The drawing under review shows one solid part. Ordinate dimensions are in mm from its lowest x, y, z. A direction names the side the tool comes from. Coordinates: 2 decimals unless noted, no trailing zeros. Loops run counter-clockwise (first coordinate to the right, second up) from the corner with the lowest first, then second, coordinate; pieces in that order, holes last. Notation, with made-up numbers: M 65.25,-13.5 L 88.25,-13.5 A17 cw 88.25,-0.5 Z; hole C 65,39 d9. An arc over 180 degrees is marked long. Put each result on its own line as item: value.
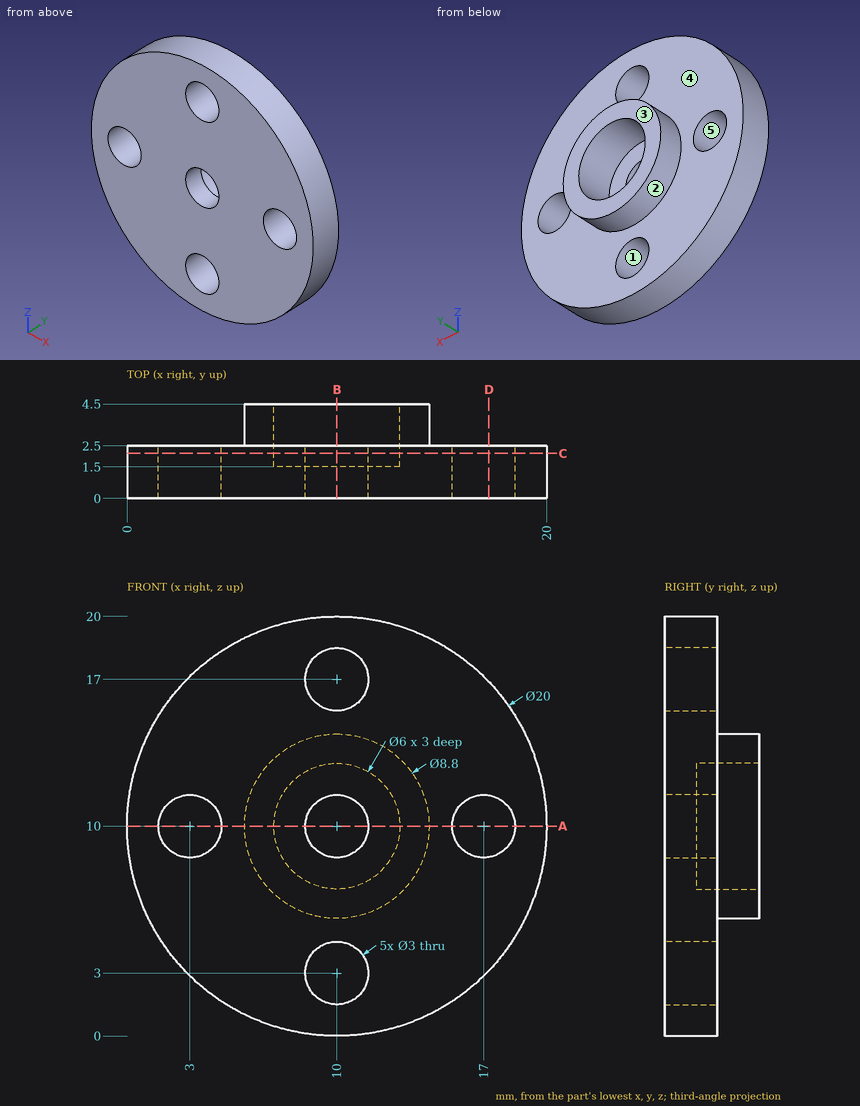
(1) Add section D-D (x = 17.25). Write out the cut boundary in (y, z).
Determined:
outline: M 0,3.11 L 2.5,3.11 L 2.5,8.52 L 0,8.52 Z; M 0,11.48 L 2.5,11.48 L 2.5,16.89 L 0,16.89 Z
(2) Tool access review of the marked faces 4 and 5: name each direction out of +Z, -Z, +X, -X, +Y, -Y from which nothing blocks a thin tool from reaching the whole face with its end or side.
Determined:
face 4: +Y
face 5: +Y, -Y
(3) For pin 1 (4 mm diameter, centred on x = 10, z = 17, fed in from +Y); pin 2 (1.5 mm diameter, centred on y = 1.5, z = 13.5, fed in from -X); pin 3 (2 mm diameter, centred on y = 1, z = 16, fed in from -X), all flat-tipped, find the tip position at first contact; note any pin that passes through.
Determined:
pin 1: stops at y = 2.5
pin 2: stops at x = 0.39
pin 3: stops at x = 1.34
(4) Draft analysis for pull direction Z (two halves, no side actions). For the marked faces 1, 2 and 3, state which applies: +Z half, -Z half, draft (parallel to the pull), parting line (faces both ways), or undercut.
Determined:
face 1: undercut
face 2: parting line
face 3: draft
(5) Wall thickness on line 1 along X through (y, z) = (0.8, 10); line 2 along X through (y, z) = (3.65, 10); line 3 along X through (y, z) = (0.5, 9.25): over which ranges is each line inside the solid? List them lowest first. Write a range as [from, to].
Determined:
line 1: x = [0, 1.5], [4.5, 8.5], [11.5, 15.5], [18.5, 20]
line 2: x = [5.6, 7], [13, 14.4]
line 3: x = [0.03, 1.7], [4.3, 8.7], [11.3, 15.7], [18.3, 19.97]
(6) Add section B-B (x = 10). Write out the cut boundary in (y, z), plus the area to 3 significant figures.
Determined:
outline: M 0,0 L 2.5,0 L 2.5,1.5 L 0,1.5 Z; M 0,4.5 L 2.5,4.5 L 2.5,5.6 L 4.5,5.6 L 4.5,7 L 1.5,7 L 1.5,8.5 L 0,8.5 Z; M 0,11.5 L 1.5,11.5 L 1.5,13 L 4.5,13 L 4.5,14.4 L 2.5,14.4 L 2.5,15.5 L 0,15.5 Z; M 0,18.5 L 2.5,18.5 L 2.5,20 L 0,20 Z
area: 30.1 mm^2
(7) Add section C-C (y = 2.15). Write out the cut boundary in (x, z), plus the area to 3 significant figures.
Determined:
outline: C 10,10 d20; hole C 3,10 d3; hole C 10,10 d6; hole C 10,3 d3; hole C 10,17 d3; hole C 17,10 d3
area: 258 mm^2
(8) Add section A-A (z = 10). Write out the cut boundary in (x, y).
Determined:
outline: M 0,0 L 1.5,0 L 1.5,2.5 L 0,2.5 Z; M 4.5,0 L 8.5,0 L 8.5,1.5 L 7,1.5 L 7,4.5 L 5.6,4.5 L 5.6,2.5 L 4.5,2.5 Z; M 11.5,0 L 15.5,0 L 15.5,2.5 L 14.4,2.5 L 14.4,4.5 L 13,4.5 L 13,1.5 L 11.5,1.5 Z; M 18.5,0 L 20,0 L 20,2.5 L 18.5,2.5 Z
